Work out the finished part from the listing and answer in its coordinate system (mm). Face numbers are marked on the shaded views. A direction names the side the tool comes from. Round coordinates to 2 decimals unless told otherwise and drop trailing zeros. Order: outer loops, then holes, each group sorted by start corner. A loop starts at its lowest first (then second) coordinate and runs counter-clockwise, first axis right, second up. Notation, with made-up numbers: (-4.5, 64) -> (13.5, 64) arc R22 ccw to (13.5, 103) -> close; hole circle Ø5 at (26, 36). An arc over 180 degrees is marked (long way). Use one line per item in the form item = value.
```python
from build123d import *

# Parameters (mm, degrees)
SKETCH1_R                 = 12.5
BOSS_EXTRUDE1_DEPTH       = 54
SKETCH2_R                 = 5
BOSS_EXTRUDE2_DEPTH       = 1.1
SKETCH3_R                 = 3.455150035
BOSS_EXTRUDE3_DEPTH       = 1.8
SKETCH4_R                 = 1.5
BOSS_EXTRUDE4_DEPTH       = 9.9
F_2_0MM_DOWEL_HOLE1_D     = 2
F_2_0MM_DOWEL_HOLE1_DEPTH = 2.8999942
F_2_0MM_DOWEL_HOLE1_TIP   = 0.600860619


with BuildPart() as part:
    # Sketch1 → Boss-Extrude1 (new body)
    with BuildSketch(Plane(origin=(0, 0, 0), x_dir=(1, 0, 0), z_dir=(0, 1, 0))):
        Circle(SKETCH1_R)
    extrude(amount=BOSS_EXTRUDE1_DEPTH)

    # Sketch2 → Boss-Extrude2 (add)
    with BuildSketch(Plane(origin=(0, 54, 0), x_dir=(1, 0, 0), z_dir=(0, 1, 0))):
        Circle(SKETCH2_R)
    extrude(amount=BOSS_EXTRUDE2_DEPTH)

    # Sketch3 → Boss-Extrude3 (add)
    with BuildSketch(Plane(origin=(0, 55.1, 0), x_dir=(1, 0, 0), z_dir=(0, 1, 0))):
        Circle(SKETCH3_R)
    extrude(amount=BOSS_EXTRUDE3_DEPTH)

    # Sketch4 → Boss-Extrude4 (add)
    with BuildSketch(Plane(origin=(0, 56.9, 0), x_dir=(1, 0, 0), z_dir=(0, 1, 0))):
        Circle(SKETCH4_R)
    extrude(amount=BOSS_EXTRUDE4_DEPTH)

    # Ø2.0mm Dowel Hole1
    with Locations(Plane(origin=(0, 54, 0), x_dir=(1, 0, 0), z_dir=(0, 1, 0))):
        with Locations((-7.361215932, -4.25), (0, 8.5), (7.361215932, -4.25)):
            Hole(F_2_0MM_DOWEL_HOLE1_D / 2, depth=F_2_0MM_DOWEL_HOLE1_DEPTH)
            with Locations((0, 0, -(F_2_0MM_DOWEL_HOLE1_DEPTH + F_2_0MM_DOWEL_HOLE1_TIP / 2))):  # 118° drill point
                Cone(0, F_2_0MM_DOWEL_HOLE1_D / 2, F_2_0MM_DOWEL_HOLE1_TIP, mode=Mode.SUBTRACT)


solid = part.part
```
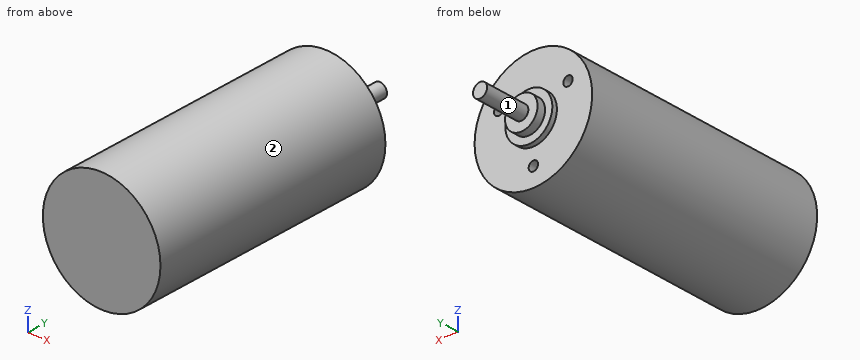
Item 1: The part is cut by section A-A, the plane z = 0. Give the vertices of the cut face in (x, y), and give its area (3 significant figures).
Findings:
outline = (-12.5, 0) -> (12.5, 0) -> (12.5, 54) -> (5, 54) -> (5, 55.1) -> (3.46, 55.1) -> (3.46, 56.9) -> (1.5, 56.9) -> (1.5, 66.8) -> (-1.5, 66.8) -> (-1.5, 56.9) -> (-3.46, 56.9) -> (-3.46, 55.1) -> (-5, 55.1) -> (-5, 54) -> (-12.5, 54) -> close
area = 1,400 mm^2
Item 2: The part is cut by section D-D, the plane z = -4.25. Give the vertices of the cut face in (x, y), and give its area (3 significant figures).
Findings:
outline = (-11.76, 0) -> (11.76, 0) -> (11.76, 54) -> (2.63, 54) -> (2.63, 55.1) -> (-2.63, 55.1) -> (-2.63, 54) -> (-11.76, 54) -> close
area = 1,280 mm^2
Item 3: Consider line 1 along Z through (x, y) = (0, 52.15); line 2 along Y through (x, z) = (9, 0.5); line 3 along X through (y, z) = (52.3, 4.25). Determine where each line is inside the solid, lowest interval first.
Findings:
line_1 = -12.5 to -9.5, -7.5 to 12.5
line_2 = 0 to 54
line_3 = -11.76 to -8.36, -6.36 to 6.36, 8.36 to 11.76
Item 4: The part is cut by section B-B, the plane x = -10. Give the vertices of the cut face in (y, z).
Findings:
outline = (0, -7.5) -> (54, -7.5) -> (54, 7.5) -> (0, 7.5) -> close
Item 5: Flat-ended cylindrical pins translate along their axes: P1, Ø4, axis at x = -3.5, z = 6.5, coming from the +Y side; P2, Ø1.8, axis at x = -7.36, z = 4.25, coming from the +Y side; P3, Ø3, axis at x = -5, y = 39, coming from the +Z side. Find the tip coordinate at first contact, or state that the pin passes through.
Findings:
P1 = 54
P2 = 51.04
P3 = 12
Item 6: The part is cut by section C-C, the plane y = 20.5. Give the vertices of the cut face in (x, z), and give its area (3 significant figures).
Findings:
outline = circle Ø25 at (0, 0)
area = 491 mm^2
Item 7: For the marked faces 1 and 2, determine the directions among +Z, -Z, +X, -X, +Y, -Y from which every point of the face is accessible in a straight line to the end or side of a thin tool.
Findings:
face_1 = +Y
face_2 = +Y, -Y
